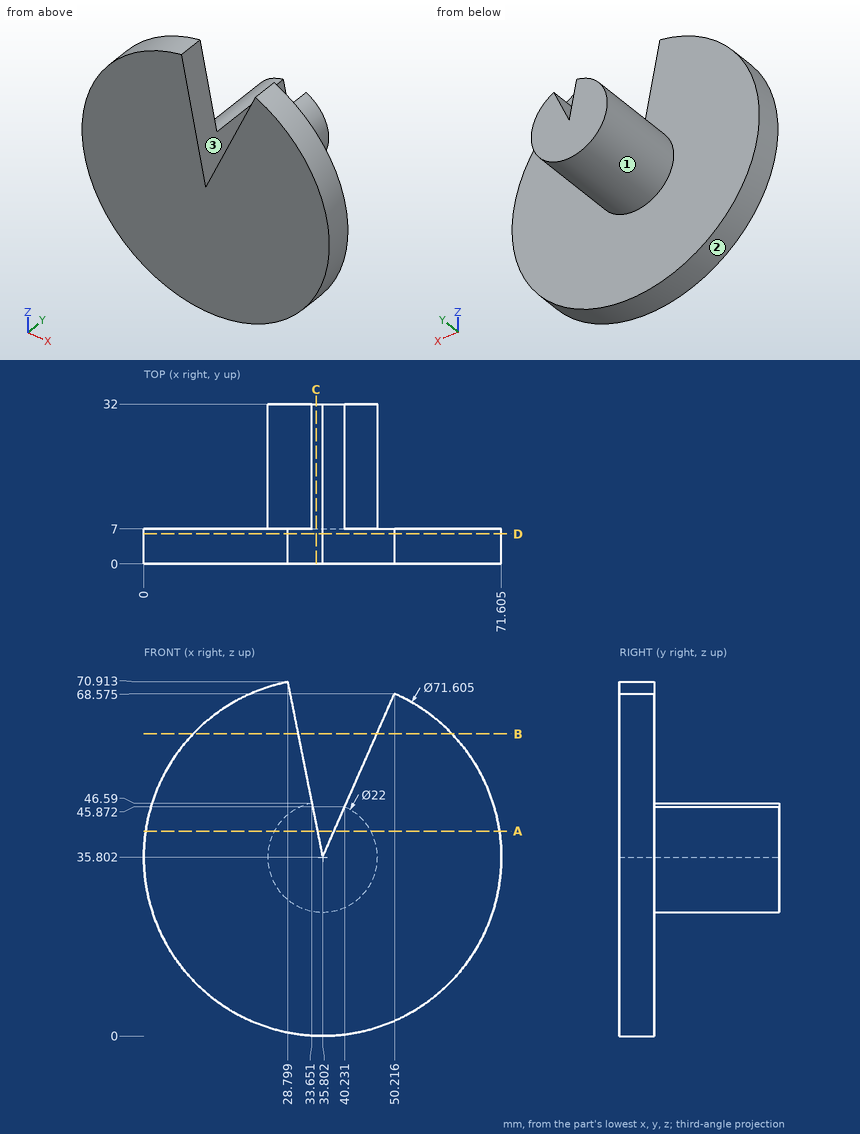
Source: three-view drawing plus pictorial views. Frame: mm from the lowest corner of the part. A direction names the side the tool comes from. Round coordinates to 2 decimals unless told otherwise and drop trailing zeros. Loops run counter-clockwise (first coordinate to the right, second up) from the corner with the lowest first, then second, coordinate; pieces in that order, holes last.
1. Ray query, L1, parallel to Y at x = 52.5, z = 34.5; L2, parallel to X at y = 2, z = 55.5 (1 decimal); L3, parallel to X at y = 4.5, z = 45. Return the intervals inside material, ascending.
2. Section query B-B on z = 60.5. Output: boundary loops of the cut face in (x, y) (1 decimal).
3. Section query A-A on z = 41. Output: boundary loops of the cut face in (x, y) (1 decimal).
4. Section query D-D on y = 6. Output: boundary loops of the cut face in (x, z) (1 decimal).
5. Access query for the marked faces 1, 2 and 3. Directions: +Z, -Z, +X, -X, +Y, -Y. A direction counts if a zero-diameter tool reaches every point of the face in a straight line with its end or side. Return the directions, or none.
6. Section query C-C on x = 34.5. Output: boundary loops of the cut face in (y, z).
7. Contact query for flat-ended pins moving along their axis: pin 1 (3 mm diameter, centred on y = 7, z = 18, fed in from +X); pin 2 (1.5 mm diameter, centred on x = 45, y = 9.5, fed in from +Z); pin 3 (10 mm diameter, centred on x = 59.5, y = 13, fed in from -Z); pin 4 (1.5 mm diameter, centred on y = 19.5, z = 36.5, fed in from +X). Output: stop coordinate, or through.
Answers below:
1. L1: y = 0 to 7
1. L2: x = 5.9 to 31.9, 44.5 to 65.7
1. L3: x = 1.2 to 33.97, 39.85 to 70.4
2. outline: (9.9, 0) - (30.9, 0) - (30.9, 7) - (9.9, 7) - close; (46.7, 0) - (61.7, 0) - (61.7, 7) - (46.7, 7) - close
3. outline: (0.4, 0) - (34.8, 0) - (34.8, 32) - (26.1, 32) - (26.1, 7) - (0.4, 7) - close; (38.1, 0) - (71.2, 0) - (71.2, 7) - (45.5, 7) - (45.5, 32) - (38.1, 32) - close
4. outline: (28.8, 70.9) arc R35.8 ccw (long way) to (50.2, 68.6) - (35.8, 35.8) - close
5. face 1: +Y
5. face 2: +Y, -Y
5. face 3: +Z, +Y, -Y
6. outline: (0, 0.02) - (7, 0.02) - (7, 24.88) - (32, 24.88) - (32, 42.33) - (0, 42.33) - close
7. pin 1: stops at x = 67.68
7. pin 2: stops at z = 42.85
7. pin 3: passes through
7. pin 4: stops at x = 46.8
